```python
from build123d import *

# Parameters (mm, degrees)
SKETCH1_R            = 22.5
BOSS_EXTRUDE1_DEPTH  = 21
CHAMFER1_SIZE        = 2
M5_CLEARANCE_HOLE1_D = 5.3


with BuildPart() as part:
    # Sketch1 → Boss-Extrude1 (new body)
    with BuildSketch(Plane(origin=(0, 0, 0), x_dir=(1, 0, 0), z_dir=(0, 1, 0))):
        with Locations(Location((0, 0, 0), (0, 0, 90))):
            Circle(SKETCH1_R)
    extrude(amount=BOSS_EXTRUDE1_DEPTH)

    # Chamfer1
    chamfer1_edges = [part.edges().sort_by_distance(p)[0] for p in [
        (0, 21, 22.5),
    ]]
    chamfer(chamfer1_edges, length=CHAMFER1_SIZE)

    # M5 Clearance Hole1 (through all)
    with Locations(Plane(origin=(0, 21, 0), x_dir=(1, 0, 0), z_dir=(0, 1, 0))):
        with Locations((-10.606601718, 10.606601718), (0, 15), (15, 0), (0, -15), (-15, 0), (10.606601718, 10.606601718), (10.606601718, -10.606601718), (-10.606601718, -10.606601718)):
            Hole(M5_CLEARANCE_HOLE1_D / 2)


solid = part.part
```
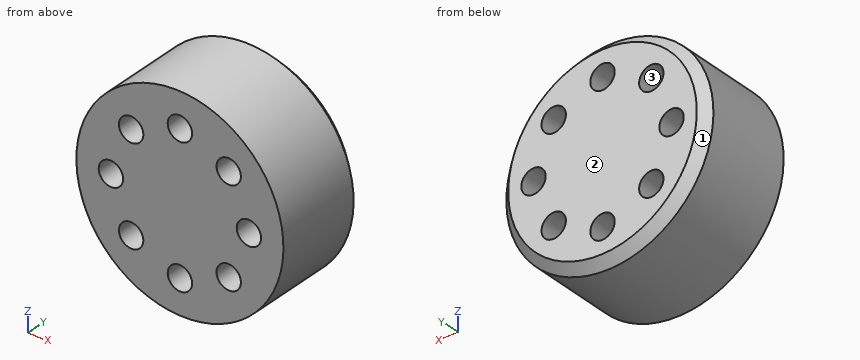
Model file for the job. Use its own axes, mm. Face numbers are marked on the shaded views. Round coordinates to 2 decimals unless told otherwise and drop trailing zeros. Order: outer loops, then holes, each group sorted by start corner. A loop starts at its lowest first (then second) coordinate and runs counter-clockwise, first axis right, second up. Notation, with made-up numbers: M -18.5,-6.5 L 25.5,-6.5 A13 ccw 25.5,-0.5 Z; hole C 56.5,-29.75 d11. An arc over 180 degrees is marked long. Use CSV: the item, a comma, the result in double quotes.
Item 1: Pin check, flat tips, straight feed: pin 1 (3 mm diameter, centred on y = 9.5, z = 2, fed in from +X); pin 2 (3 mm diameter, centred on y = 16, z = 10, fed in from -X); pin 3 (3 mm diameter, centred on x = -10.61, z = -10.61, fed in from +Y); pin 4 (3 mm diameter, centred on x = -17.5, z = -15.5, fed in from +Y). Stop position of each tip, or through.
Worked answers:
pin 1,"x = 22.49"
pin 2,"x = -20.83"
pin 3,"through"
pin 4,"y = 19.62"
Item 2: Pull direction X, two halves, no side cores. Call the marked faces 1, 2 and 3: released by +X, released by -X, zero draft, split by the parting line, or undercut.
Worked answers:
face 1,"split by the parting line"
face 2,"zero draft"
face 3,"undercut"
Item 3: Saw through at A-A (x = 0). List the corners of the cut face in (y, z), plus the area to 3 significant figures.
Worked answers:
outline,"M 0,-22.5 L 19,-22.5 L 21,-20.5 L 21,-17.65 L 0,-17.65 Z; M 0,-12.35 L 21,-12.35 L 21,12.35 L 0,12.35 Z; M 0,17.65 L 21,17.65 L 21,20.5 L 19,22.5 L 0,22.5 Z"
area,"718 mm²"
Item 4: Probe probe 1 along X at (y, z) = (16, 1.5); probe 2 along Z at (x, y) = (-2, 12.25); probe 3 along Z at (x, y) = (1, 19.75). List the from-to ranges inside material, lowest first.
Worked answers:
probe 1,"-22.45 to -17.18, -12.82 to 12.82, 17.18 to 22.45"
probe 2,"-22.41 to -16.74, -13.26 to 13.26, 16.74 to 22.41"
probe 3,"-21.73 to -17.45, -12.55 to 12.55, 17.45 to 21.73"
Item 5: Saw through at B-B (y = 12.25). State how many separate pieces and enclosed holes the cut face has, plus the area to 3 significant figures.
Worked answers:
separate pieces,"1"
enclosed holes,"8"
area,"1,410 mm²"
